```python
from build123d import *

# Parameters (mm, degrees)
SKETCH_1_R               = 1.5
SKETCH_1_R_2             = 29.8
EXTRUDE_1_DEPTH          = 3
CHAMFER_1_SIZE           = 0.5
CUT_EXTRUDE_1_DEPTH      = 302.180394913
CUT_EXTRUDE_1_DEPTH_BACK = 302.180394913
SKETCH_2_R               = 1.5
CUT_EXTRUDE_2_DEPTH      = 302.180394913
CUT_EXTRUDE_2_DEPTH_BACK = 302.180394913
SKETCH_3_R               = 1.5


with BuildPart() as part:
    # 草图1 → 凸台-拉伸1 (new body)
    with BuildSketch(Plane.XZ.offset(-78.025173071)):
        with BuildLine():
            Line((-212.561517714, -108.249692404), (-212.240178336, -124.096924988))
            ThreePointArc((-212.240178336, -124.096924988), (-212.661273384, -127.177841531), (-214.008389255, -129.980455778))
            ThreePointArc((-214.008389255, -129.980455778), (-174.628775953, -203.200190572), (-138.249712047, -128.44427297))
            ThreePointArc((-138.249712047, -128.44427297), (-139.709332875, -125.698571817), (-140.25497588, -122.637258129))
            Line((-140.25497588, -122.637258129), (-140.576315258, -106.790025545))
            ThreePointArc((-140.576315258, -106.790025545), (-141.497820174, -104.686954783), (-143.636518146, -103.851461562))
            Line((-143.636518146, -103.851461562), (-209.622953731, -105.189489516))
            ThreePointArc((-209.622953731, -105.189489516), (-211.726024493, -106.110994432), (-212.561517714, -108.249692404))
        make_face()
        with Locations((-136.648445194, -139.453062321)):
            Circle(SKETCH_1_R, mode=Mode.SUBTRACT)
        with Locations((-175.575532096, -156.509788424)):
            Circle(SKETCH_1_R_2, mode=Mode.SUBTRACT)
        with Locations((-135.988998284, -171.974468852)):
            Circle(SKETCH_1_R, mode=Mode.SUBTRACT)
        with Locations((-191.040212525, -196.096322235)):
            Circle(SKETCH_1_R, mode=Mode.SUBTRACT)
        with Locations((-215.162065908, -141.045107995)):
            Circle(SKETCH_1_R, mode=Mode.SUBTRACT)
        with Locations((-192.632258198, -117.582701522)):
            Circle(SKETCH_1_R, mode=Mode.SUBTRACT)
        with Locations((-160.110851668, -116.923254612)):
            Circle(SKETCH_1_R, mode=Mode.SUBTRACT)
        with Locations((-214.502618998, -173.566514526)):
            Circle(SKETCH_1_R, mode=Mode.SUBTRACT)
        with Locations((-158.518805994, -195.436875326)):
            Circle(SKETCH_1_R, mode=Mode.SUBTRACT)
    extrude(amount=EXTRUDE_1_DEPTH)

    # 倒角1
    chamfer_1_edges = [part.edges().sort_by_distance(p)[0] for p in [
        (-212.400848023, 78.025173077, -116.173308696),
        (-211.72602449, 78.025173077, -106.110994432),
        (-176.629735936, 78.025173076, -104.520475539),
        (-141.497820172, 78.025173075, -104.686954784),
        (-211.72602449, 75.025173077, -106.110994432),
        (-212.400848023, 75.025173077, -116.173308696),
        (-212.661273381, 75.025173077, -127.177841532),
        (-174.628775951, 75.025173075, -203.200190573),
        (-205.375532094, 78.025173077, -156.509788424),
        (-205.375532094, 75.025173077, -156.509788424),
        (-139.709332873, 75.025173075, -125.698571818),
        (-140.415645567, 75.025173075, -114.713641837),
        (-141.497820172, 75.025173075, -104.686954784),
        (-140.415645566, 78.025173075, -114.713641837),
        (-176.629735936, 75.025173076, -104.520475539),
        (-139.709332873, 78.025173075, -125.698571818),
        (-174.62877595, 78.025173075, -203.200190573),
        (-212.661273381, 78.025173077, -127.177841532),
    ]]
    chamfer(chamfer_1_edges, length=CHAMFER_1_SIZE)

    # 草图2 → 切除-拉伸1 (cut, two sides: drawn at the far end of the back side and taken through both)
    with BuildSketch(Plane(origin=(2e-09, 78.025173071, -1e-09), x_dir=(1.0, -3.1446611841336594e-11, 0), z_dir=(3.1446611841336594e-11, 1.0, -6.574611909583631e-12)).offset(-CUT_EXTRUDE_1_DEPTH_BACK)):
        with Locations(Location((-200.041202679, 114.05266186, 0), (0, 0, 180))):
            Circle(SKETCH_2_R)
    extrude(amount=CUT_EXTRUDE_1_DEPTH + CUT_EXTRUDE_1_DEPTH_BACK, mode=Mode.SUBTRACT)

    # 草图3 → 切除-拉伸2 (cut, two sides: drawn at the far end of the back side and taken through both)
    with BuildSketch(Plane(origin=(2e-09, 78.025173071, -1e-09), x_dir=(1.0, -3.1446611841336594e-11, 0), z_dir=(3.1446611841336594e-11, 1.0, -6.574611909583631e-12)).offset(-CUT_EXTRUDE_2_DEPTH_BACK)):
        with Locations(Location((-152.851097985, 113.09577309, 0), (0, 0, 180))):
            Circle(SKETCH_3_R)
    extrude(amount=CUT_EXTRUDE_2_DEPTH + CUT_EXTRUDE_2_DEPTH_BACK, mode=Mode.SUBTRACT)


solid = part.part
```
Part model, mm, in its own coordinate system. Coordinates: 2 decimals unless noted, no trailing zeros. Write item = value, one per line. Start each with the question number.
Item 1: Wall check: L1, parallel to X at y = 76.25, z = -138.5; L2, parallel to X at y = 76.5, z = -114; L3, parallel to X at y = 75.75, z = -156. Give the ranges that are in metal, low to high. Write a range as from..to.
Item 2: Flat gauge pin, fed straight in: pin 1 Ø1.5 at (x, y) = (-209, 77) entering from +Z. Where does the tip first touch, or does it go through?
Item 3: Mould opens along X. For faces 1 (the cylindrical face through (-161.61, 76.55, -116.86)), 2 (the cylindrical face through (-176.064, 76.539, -203.207)), 3 (the cylindrical face through (-211.703, 76.539, -106.087)), 4 (the flat face through (-197, 78.025, -131)) say: released by +X, released by -X, zero draft, split by the parting line, or undercut.
Item 4: Cut at A-A, the plane y = 76.45. State how many separate pieces and enclosed holes the cut face has, and give its area (3 significant figures).
The answers:
q1.L1 = -218.66..-199.32, -151.83..-137.81, -135.49..-132.49
q1.L2 = -212.44..-201.54, -198.54..-154.05, -151.65..-140.43
q1.L3 = -222.27..-205.37, -145.78..-128.88
q2.pin_1 = -105.16
q3.face_1 = undercut
q3.face_2 = split by the parting line
q3.face_3 = released by -X
q3.face_4 = zero draft
q4.separate_pieces = 1
q4.enclosed_holes = 11
q4.area = 4,740 mm2
